Check sheet for the modelled part. Datum: model origin and axes. Units: mm. A direction names the side the tool comes from. Round coordinates to 2 decimals unless told otherwise and drop trailing zeros. Loops run counter-clockwise (first coordinate to the right, second up) from the corner with the lowest first, then second, coordinate; pieces in that order, holes last. Notation, with made-up numbers: (16.5, -35.5) -> (58.5, -35.5) arc R23 cw to (58.5, -5.5) -> close; hole circle Ø9 at (-25, -30). An arc over 180 degrees is marked (long way). Use one line per item in the form item = value. Start each with the question number.
(1) Go/stop test with flat-tipped pins: pin 1 (3 mm diameter, centred on y = 27, z = 4, fed in from +X); pin 2 (4 mm diameter, centred on x = -33.53, y = -6.68, fed in from -Z); pin 3 (19.5 mm diameter, centred on x = -12.5, y = -5, fed in from +Z); pin 4 (1 mm diameter, centred on y = -8, z = 4, fed in from +X). Record where each tip stops, or that it passes through.
(2) Sectioned sample at A-A (y = 0). Record the cut outline in (x, z), and give its area (3 significant figures).
(3) Sectioned sample at C-C (y = 28). Record the cut outline in (x, z).
(4) Sectioned sample at D-D (z = 1.95). Record the cut outline in (x, y), and give its area (3 significant figures).
(5) Set-up check for faces 1 (the cylindrical face through (11.85, 33.75, 2.58)), 2 (the flat face through (-12.2, 24.3, 1.016)): record each of +Z, -Z, +X, -X, +Y, -Y from which the full face is reachable in a straight line by a thin tool's end or side.
(6) Draft check along X on faces 3 (the cylindrical face through (-25.82, -19.8, 3.09)), 4 (the cylindrical face through (-8.436, -37.987, 4.331)), 5 (the flat face through (9, -27, 0)). Enter one of: released by +X, released by -X, zero draft, split by the parting line, or undercut.
(7) Material ranges on probe 1 along Y at (x, z) = (23, 0.6); probe 2 along Y at (x, z) = (0, 0.6); probe 3 along Y at (x, z) = (0, 2.9), recorded low to high. Write a range as [from, to].
from build123d import *

# Parameters (mm, degrees)
F0_R     = 38.9128
F0_R_2   = 1.6256
F0_R_3   = 32.5374
F1_DEPTH = 5.2324
F2_R     = 32.5374
F2_R_2   = 26.9875
F3_DEPTH = 1.016
F4_R     = 40.9448
F4_R_2   = 38.9128
F5_DEPTH = 3.4544


with BuildPart() as f1:
    # F0 (on Top) → F1 (new body)
    with BuildSketch(Plane.XY):
        Circle(F0_R)
        with Locations((-33.529478, -6.679878)):
            Circle(F0_R_2, mode=Mode.SUBTRACT)
        with Locations((22.549683, -25.697441)):
            Circle(F0_R_2, mode=Mode.SUBTRACT)
        Circle(F0_R_3, mode=Mode.SUBTRACT)
        with Locations((10.979795, 32.377319)):
            Circle(F0_R_2, mode=Mode.SUBTRACT)
    extrude(amount=F1_DEPTH)

    # F2 (on Top) → F3 (join)
    with BuildSketch(Plane.XY):
        Circle(F2_R)
        Circle(F2_R_2, mode=Mode.SUBTRACT)
    extrude(amount=F3_DEPTH)

    # F4 (on Top) → F5 (join)
    with BuildSketch(Plane.XY):
        Circle(F4_R)
        Circle(F4_R_2, mode=Mode.SUBTRACT)
    extrude(amount=F5_DEPTH)


solid = f1.part
Checks:
q1.pin_1 = 31.95
q1.pin_2 = 0
q1.pin_3 = through
q1.pin_4 = 38.18
q2.outline = (-40.94, 0) -> (-26.99, 0) -> (-26.99, 1.02) -> (-32.54, 1.02) -> (-32.54, 5.23) -> (-38.91, 5.23) -> (-38.91, 3.45) -> (-40.94, 3.45) -> close; (26.99, 0) -> (40.94, 0) -> (40.94, 3.45) -> (38.91, 3.45) -> (38.91, 5.23) -> (32.54, 5.23) -> (32.54, 1.02) -> (26.99, 1.02) -> close
q2.area = 92.0 mm2
q3.outline = (-29.87, 0) -> (29.87, 0) -> (29.87, 3.45) -> (27.02, 3.45) -> (27.02, 5.23) -> (16.57, 5.23) -> (16.57, 1.02) -> (-16.57, 1.02) -> (-16.57, 5.23) -> (-27.02, 5.23) -> (-27.02, 3.45) -> (-29.87, 3.45) -> close
q4.outline = circle Ø81.89 at (0, 0); hole circle Ø3.25 at (-33.53, -6.68); hole circle Ø65.07 at (0, 0); hole circle Ø3.25 at (10.98, 32.38); hole circle Ø3.25 at (22.55, -25.7)
q4.area = 1,920 mm2
q5.face_1 = +Z, -Z
q5.face_2 = +Z
q6.face_3 = undercut
q6.face_4 = split by the parting line
q6.face_5 = zero draft
q7.probe_1 = [-33.87, -27.26], [-24.14, -14.12], [14.12, 33.87]
q7.probe_2 = [-40.94, -26.99], [26.99, 40.94]
q7.probe_3 = [-40.94, -32.54], [32.54, 40.94]
